Geometry: final body of the model. Coordinates: model frame, mm. A direction names the side the tool comes from. Give positions to 0.01 mm unless a question says otherwise; leave off trailing zeros. Write each loop counter-clockwise with the first axis right and the second up, starting at its lowest first coordinate (ties: lowest second). Pieces come first, ordered by that corner, then holes. Notation, with made-up numbers: (45.25, 73.5) -> (54.25, 73.5) arc R25 cw to (54.25, 111.5) -> close; hole circle Ø2 at (41.25, 79). An arc over 180 degrees is marked (long way). Answer in a Markdown table with one row per item. Add a question column.
Item 1: Section query A-A on x = 0. Output: boundary loops of the cut face in (y, z).
Item 2: Material intervals for probe 1 along X at (y, z) = (27, 0); probe 2 along Y at (x, z) = (-30.5, -17.5), sorted ascending. Write a range as from..to.
Item 3: Section query D-D on y = 25.5. Output: boundary loops of the cut face in (x, z) (3 decimals).
Item 4: Section query B-B on z = 0. Output: boundary loops of the cut face in (x, y), plus the area to 3 significant figures.
Item 5: First-contact query: P1, Ø5, axis at x = -29.5, z = 27.5, coming from the +Y side; P2, Ø1, axis at x = -8.5, y = 7, coming from the +Z side; P3, Ø11, axis at x = -28.28, z = -28.28, coming from the -Y side; P4, Ø4.5, axis at x = 28.28, z = 28.28, coming from the +Y side. Flat tips, straight axial feed; report the tip coordinate or a pass-through.
Item 6: Draft query along Z for faces 1 (the flat face through (-30, 35, 26)), 2 (the flat face through (-1, 40, 10)), 3 (the cylindrical face through (-14.985, 10.14, -0.66)). Return one class per face: +Z half, -Z half, draft (parallel to the pull), parting line (faces both ways), or undercut.
Item 7: Access query for faces 4 (the flat face through (-3, 0, 3)), 5 (the flat face through (-10, 20, -12)), 6 (the cylindrical face through (-32.934, 37.535, 29.749)). Directions: +Z, -Z, +X, -X, +Y, -Y. A direction counts if a zero-diameter tool reaches every point of the face in a straight line with its end or side. Return the directions, or none.
Item 8: Section query C-C on x = -27. Output: boundary loops of the cut face in (y, z).
```python
from build123d import *

# Parameters (mm, degrees)
F3_D           = 5.25
F3_CBORE_D     = 9.75
F3_CBORE_DEPTH = 5


with BuildPart() as f1:
    # F0 (on Top) → F1 (revolve)
    with BuildSketch(Plane.XY):
        Polygon((50, 20), (50, 40), (3.75, 40), (3.75, 0), (15, 0), (15, 20), align=None)
    revolve(axis=Axis((0, 20, 0), (0, 1, 0)))

    # F3 (through all)
    with Locations(Plane(origin=(0, 40, 0), x_dir=(-1, 0, 0), z_dir=(0, 1, 0))):
        with Locations((-28.2842712475, 28.2842712475), (28.2842712475, 28.2842712475), (-28.2842712475, -28.2842712475), (28.2842712475, -28.2842712475)):
            CounterBoreHole(F3_D / 2, F3_CBORE_D / 2, F3_CBORE_DEPTH)


solid = f1.part
```
Findings below:
| question | item | result |
|---|---|---|
| 1 | outline | (0, -15) -> (20, -15) -> (20, -50) -> (40, -50) -> (40, -3.75) -> (0, -3.75) -> close; (0, 3.75) -> (40, 3.75) -> (40, 50) -> (20, 50) -> (20, 15) -> (0, 15) -> close |
| 2 | probe 1 | x = -50..-3.75, 3.75..50 |
| 2 | probe 2 | y = 20..40 |
| 3 | outline | circle Ø100 at (0, 0); hole circle Ø5.25 at (-28.284, -28.284); hole circle Ø5.25 at (-28.284, 28.284); hole circle Ø7.5 at (0, 0); hole circle Ø5.25 at (28.284, -28.284); hole circle Ø5.25 at (28.284, 28.284) |
| 4 | outline | (-50, 20) -> (-15, 20) -> (-15, 0) -> (-3.75, 0) -> (-3.75, 40) -> (-50, 40) -> close; (3.75, 0) -> (15, 0) -> (15, 20) -> (50, 20) -> (50, 40) -> (3.75, 40) -> close |
| 4 | area | 2,300 mm^2 |
| 5 | P1 | stops at y = 35 |
| 5 | P2 | stops at z = 12.69 |
| 5 | P3 | stops at y = 20 |
| 5 | P4 | passes through |
| 6 | face 1 | undercut |
| 6 | face 2 | draft |
| 6 | face 3 | parting line |
| 7 | face 4 | +Z, -Z, +X, -X, -Y |
| 7 | face 5 | -Y |
| 7 | face 6 | +Y |
| 8 | outline | (20, -42.08) -> (40, -42.08) -> (40, -32.99) -> (35, -32.99) -> (35, -30.57) -> (20, -30.57) -> close; (20, -25.99) -> (35, -25.99) -> (35, -23.58) -> (40, -23.58) -> (40, 23.58) -> (35, 23.58) -> (35, 25.99) -> (20, 25.99) -> close; (20, 30.57) -> (35, 30.57) -> (35, 32.99) -> (40, 32.99) -> (40, 42.08) -> (20, 42.08) -> close |
